CAD build for the part. Positions are in the model's coordinates, mm. A direction names the side the tool comes from. Give positions to 0.01 mm unless a question says otherwise; leave off trailing zeros. Loops run counter-clockwise (first coordinate to the right, second up) from the corner with the lowest first, then second, coordinate; pieces in that order, holes last.
Item 1: Saw through at C-C on x = 15. Give the cut face in (y, z), plus the area to 3 significant figures.
Item 2: Saw through at A-A on z = -12.5. Give the cut face in (x, y) (3 decimals), plus the area to 3 significant figures.
Item 3: Drop flat-ended pins along their axis: P1, Ø1, axis at x = -64.5, y = 1.5, coming from the +Z side; P2, Ø2.5, axis at x = -77, z = 13.75, coming from the -Y side; P3, Ø0.8, axis at y = 0.5, z = 30, coming from the +X side. Give the stop position or say it passes through.
Item 4: Probe probe 1 along Z at (x, y) = (-77, 0.55) (3 decimals); probe 2 along X at (y, z) = (0.75, 7); probe 3 along X at (y, z) = (1.8, 1). List the from-to ranges inside material, lowest first.
Item 5: Saw through at D-D on y = 1.3. Give the number of separate pieces and of enclosed holes in the cut face, plus the area to 3 significant figures.
Item 6: Mould opens along X. For faces 3 (the cylindrical face through (-75.545, 0.986, -6.708)), 4 (the flat face through (-1, 0, -9)) say: released by +X, released by -X, zero draft, split by the parting line, or undercut.
Item 7: Saw through at B-B on z = 17. Give the cut face in (x, y).
Item 8: Which spindle directions (+Z, -Z, +X, -X, +Y, -Y) get a long thin tool onto all of the face, cutting with end or side? Do faces 1 (the cylindrical face through (78.41, 0.99, 14.33)), 2 (the flat face through (-35.1, 1, -3.4)). Say none if no direction does.
from build123d import *

# Parameters (mm, degrees)
SKETCH_1_W          = 160
SKETCH_1_H          = 49
SKETCH_1_R          = 1.525
SKETCH_1_R_2        = 2.025
EXTRUDE_1_DEPTH     = 2
SKETCH_2_W          = 80
SKETCH_2_H          = 33
SKETCH_2_W_2        = 18
CUT_EXTRUDE_1_DEPTH = 10
CHAMFER_1_SIZE      = 10
FILLET_1_R          = 2
SKETCH_3_W          = 30
SKETCH_3_H          = 5
CUT_EXTRUDE_2_DEPTH = 10
SKETCH_4_W          = 25
SKETCH_4_H          = 5
EXTRUDE_2_DEPTH     = 2
FILLET_2_R          = 2
SKETCH_5_W          = 80
SKETCH_5_H          = 18.828427125
CUT_EXTRUDE_3_DEPTH = 10
FILLET_3_R          = 2


with BuildPart() as part:
    # 草图1 → 凸台-拉伸1 (new body)
    with BuildSketch(Plane(origin=(0, 0, 0), x_dir=(1, 0, 0), z_dir=(0, 1, 0))):
        with Locations((0, -8)):
            Rectangle(SKETCH_1_W, SKETCH_1_H)
        with Locations((-77, -13.75)):
            Circle(SKETCH_1_R, mode=Mode.SUBTRACT)
        with Locations((-77, 6.25)):
            Circle(SKETCH_1_R, mode=Mode.SUBTRACT)
        with Locations((77, 6.25)):
            Circle(SKETCH_1_R, mode=Mode.SUBTRACT)
        with Locations((77, -13.75)):
            Circle(SKETCH_1_R, mode=Mode.SUBTRACT)
        with Locations((-47.5, 12.5)):
            Circle(SKETCH_1_R_2, mode=Mode.SUBTRACT)
        with Locations((-47.5, -12.5)):
            Circle(SKETCH_1_R_2, mode=Mode.SUBTRACT)
        with Locations((47.5, 12.5)):
            Circle(SKETCH_1_R_2, mode=Mode.SUBTRACT)
        with Locations((47.5, -12.5)):
            Circle(SKETCH_1_R_2, mode=Mode.SUBTRACT)
    extrude(amount=EXTRUDE_1_DEPTH)

    # 草图2 → 切除-拉伸1 (cut)
    with BuildSketch(Plane(origin=(0, 2, 0), x_dir=(1, 0, 0), z_dir=(0, 1, 0))):
        with Locations((0, -8)):
            Rectangle(SKETCH_2_W, SKETCH_2_H)
        with Locations((64, -8)):
            Rectangle(SKETCH_2_W_2, SKETCH_2_H)
        with Locations((-64, -8)):
            Rectangle(SKETCH_2_W_2, SKETCH_2_H)
    extrude(amount=-CUT_EXTRUDE_1_DEPTH, mode=Mode.SUBTRACT)

    # 倒角1
    chamfer_1_edges = [part.edges().sort_by_distance(p)[0] for p in [
        (40, 1, -8.5),
        (40, 1, 24.5),
        (-40, 1, 24.5),
        (-40, 1, -8.5),
    ]]
    chamfer(chamfer_1_edges, length=CHAMFER_1_SIZE)

    # 圆角1
    fillet_1_edges = [part.edges().sort_by_distance(p)[0] for p in [
        (30, 1, 24.5),
        (-30, 1, 24.5),
        (-40, 1, 1.5),
        (-40, 1, 14.5),
        (40, 1, 1.5),
        (40, 1, 14.5),
        (-30, 1, -8.5),
        (30, 1, -8.5),
        (73, 1, -8.5),
        (73, 1, 24.5),
        (55, 1, 24.5),
        (55, 1, -8.5),
        (-73, 1, 24.5),
        (-73, 1, -8.5),
        (-55, 1, -8.5),
        (-55, 1, 24.5),
    ]]
    fillet(fillet_1_edges, radius=FILLET_1_R)

    # 草图3 → 切除-拉伸2 (cut)
    with BuildSketch(Plane.XZ):
        with Locations((-65, 30)):
            Rectangle(SKETCH_3_W, SKETCH_3_H)
        with Locations((65, 30)):
            Rectangle(SKETCH_3_W, SKETCH_3_H)
    extrude(amount=-CUT_EXTRUDE_2_DEPTH, mode=Mode.SUBTRACT)

    # 草图4 → 凸台-拉伸2 (add)
    with BuildSketch(Plane.XZ):
        with Locations((-67.5, 25)):
            Rectangle(SKETCH_4_W, SKETCH_4_H)
        with Locations((67.5, 25)):
            Rectangle(SKETCH_4_W, SKETCH_4_H)
    extrude(amount=-EXTRUDE_2_DEPTH)

    # 圆角2
    fillet_2_edges = [part.edges().sort_by_distance(p)[0] for p in [
        (50, 1, 32.5),
        (-50, 1, 32.5),
        (-50, 1, 27.5),
        (-80, 1, 27.5),
        (80, 1, 27.5),
        (50, 1, 27.5),
        (-80, 1, -16.5),
        (80, 1, -16.5),
    ]]
    fillet(fillet_2_edges, radius=FILLET_2_R)

    # 草图5 → 切除-拉伸3 (cut)
    with BuildSketch(Plane.XZ):
        with Locations((0, 23.085786438)):
            Rectangle(SKETCH_5_W, SKETCH_5_H)
    extrude(amount=-CUT_EXTRUDE_3_DEPTH, mode=Mode.SUBTRACT)

    # 圆角3
    fillet_3_edges = [part.edges().sort_by_distance(p)[0] for p in [
        (-40, 1, 32.5),
        (40, 1, 32.5),
    ]]
    fillet(fillet_3_edges, radius=FILLET_3_R)


solid = part.part
Results below:
1. outline: (0, -16.5) - (2, -16.5) - (2, -8.5) - (0, -8.5) - close
1. area: 16.0 mm2
2. outline: (-80, 0) - (-49.525, 0) - (-49.525, 2) - (-80, 2) - close; (-45.475, 0) - (45.475, 0) - (45.475, 2) - (-45.475, 2) - close; (49.525, 0) - (80, 0) - (80, 2) - (49.525, 2) - close
2. area: 304 mm2
3. P1: stops at z = 27.5
3. P2: passes through
3. P3: stops at x = 50
4. probe 1: z = -16.5 to -7.775, -4.725 to 12.225, 15.275 to 27.5
4. probe 2: x = -80 to -73, -55 to -40, 40 to 55, 73 to 80
4. probe 3: x = -80 to -73, -55 to -39.5, 39.5 to 55, 73 to 80
5. separate pieces: 1
5. enclosed holes: 10
5. area: 3,160 mm2
6. face 3: undercut
6. face 4: zero draft
7. outline: (-80, 0) - (-73, 0) - (-73, 2) - (-80, 2) - close; (-55, 0) - (-40, 0) - (-40, 2) - (-55, 2) - close; (40, 0) - (55, 0) - (55, 2) - (40, 2) - close; (73, 0) - (80, 0) - (80, 2) - (73, 2) - close
8. face 1: +Y, -Y
8. face 2: +Z, +Y, -Y
